```python
from build123d import *

# Parameters (mm, degrees)
SKETCH_1_R          = 5.9
EXTRUDE_1_DEPTH     = 25
SKETCH_2_R          = 2.5
CUT_EXTRUDE_2_DEPTH = 10
SKETCH_3_R          = 1.5
CUT_EXTRUDE_3_DEPTH = 15
SKETCH_5_R          = 1.5
CUT_EXTRUDE_4_DEPTH = 6
CUT_EXTRUDE_START   = -9
SKETCH_6_R          = 5.9
SKETCH_6_R_2        = 4
CUT_EXTRUDE_5_DEPTH = 9


with BuildPart() as part:
    # Эскиз1 → Вытянуть1 (new body)
    with BuildSketch(Plane.XY):
        Circle(SKETCH_1_R)
    extrude(amount=EXTRUDE_1_DEPTH)

    # Эскиз2 → Вытянуть2 (cut)
    with BuildSketch(Plane.XY.offset(25)):
        Circle(SKETCH_2_R)
    extrude(amount=-CUT_EXTRUDE_2_DEPTH, mode=Mode.SUBTRACT)

    # Эскиз3 → Вытянуть3 (cut)
    with BuildSketch(Plane(origin=(0, 0, 0), x_dir=(-1, 0, 0), z_dir=(0, 0, -1))):
        Circle(SKETCH_3_R)
    extrude(amount=-CUT_EXTRUDE_3_DEPTH, mode=Mode.SUBTRACT)

    # Эскиз5 → Вытянуть4 (cut)
    with BuildSketch(Plane(origin=(0, 7, 0), x_dir=(-1, 0, 0), z_dir=(0, 1, 0))):
        with Locations(Location((0, 4.063182322, 0), (0, 0, 90))):
            Circle(SKETCH_5_R)
        with Locations(Location((0, 12.352632006, 0), (0, 0, 90))):
            Circle(SKETCH_5_R)
    extrude(amount=-CUT_EXTRUDE_4_DEPTH, mode=Mode.SUBTRACT)

    # Эскиз6 → Вытянуть5 (cut)
    with BuildSketch(Plane.XY.offset(25).offset(CUT_EXTRUDE_START)):
        Circle(SKETCH_6_R)
        Circle(SKETCH_6_R_2, mode=Mode.SUBTRACT)
    extrude(amount=CUT_EXTRUDE_5_DEPTH, mode=Mode.SUBTRACT)


solid = part.part
```
The model under review builds one solid part; all positions refer to its coordinate system, in mm. A direction names the side the tool comes from. Round coordinates to 2 decimals unless told otherwise and drop trailing zeros. Write each loop counter-clockwise with the first axis right and the second up, starting at its lowest first coordinate (ties: lowest second). Pieces come first, ordered by that corner, then holes.
(1) We need section A-A on y = -0.5. Give the boundary of the cut face in (x, z).
(2) Mouldability with a two-part tool opening along X and no side actions: class faces 1 (the flat face through (0, -2, 15)), 2 (the cylindrical face through (-1.28, -5.76, 7.89)), 3 (the flat face through (1.2, -1.2, 0)) as +X half, -X half, draft (parallel to the pull), parting line (faces both ways), or undercut.
(3) Insertion check: pin 1 (4 mm diameter, centred on y = 3, z = 10, fed in from -X); pin 2 (5 mm diameter, centred on y = 4, z = 4.5, fed in from +X); pin 3 (1.5 mm diameter, centred on y = 3.5, z = 20, fed in from -X). Each pin has a flat end and moves straight along its axis. Give the tip position at first contact, or say it passes through.
(4) We need section C-C on z = 10.5. Give the boundary of the cut face in (x, y).
(5) Wall thickness on L1, parallel to Y at x = 0, z = 9; L2, parallel to Z at x = -1, y = 3.5; L3, parallel to Z at x = 0.75, y = 5.5: over which ranges is each line inside the solid? List them lowest first.
(6) Machinability: for faces 4 (the cylindrical face through (0.066, 3.487, 2.565)), 5 (the cylindrical face through (0.325, -1.464, 7.395)), 6 (the cylindrical face through (-0.54, -2.44, 20.07)), which of the approach directions +Z, -Z, +X, -X, +Y, -Y give a long, thin tool a straight path to every point of the face, cutting with its end or side? Answer none if there is none.
(7) We need section D-D on y = -3. Give the boundary of the cut face in (x, z).
(8) We need section B-B on x = 0. Give the boundary of the cut face in (y, z), and give its area (3 significant figures).
Findings below:
1. outline: (-5.88, 0) - (-1.41, 0) - (-1.41, 15) - (-2.45, 15) - (-2.45, 25) - (-3.97, 25) - (-3.97, 16) - (-5.88, 16) - close; (1.41, 0) - (5.88, 0) - (5.88, 16) - (3.97, 16) - (3.97, 25) - (2.45, 25) - (2.45, 15) - (1.41, 15) - close
2. face 1: undercut
2. face 2: parting line
2. face 3: draft
3. pin 1: stops at x = -5.81
3. pin 2: stops at x = 5.71
3. pin 3: stops at x = -2.9
4. outline: circle Ø11.8 at (0, 0); hole circle Ø3 at (0, 0)
5. L1: y = -5.9 to -1.5, 1.5 to 5.9
5. L2: z = 0 to 2.95, 5.18 to 11.23, 13.47 to 25
5. L3: z = 0 to 2.76, 5.36 to 11.05, 13.65 to 16
6. face 4: +Y
6. face 5: +Z, -Z
6. face 6: +Z
7. outline: (-5.08, 0) - (5.08, 0) - (5.08, 16) - (2.65, 16) - (2.65, 25) - (-2.65, 25) - (-2.65, 16) - (-5.08, 16) - close
8. outline: (-5.9, 0) - (-1.5, 0) - (-1.5, 15) - (-2.5, 15) - (-2.5, 25) - (-4, 25) - (-4, 16) - (-5.9, 16) - close; (1.5, 0) - (5.9, 0) - (5.9, 2.56) - (1.5, 2.56) - close; (1.5, 5.56) - (5.9, 5.56) - (5.9, 10.85) - (1.5, 10.85) - close; (1.5, 13.85) - (5.9, 13.85) - (5.9, 16) - (4, 16) - (4, 25) - (2.5, 25) - (2.5, 15) - (1.5, 15) - close
8. area: 139 mm2
